Here's how the part is built. I have some questions about the finished solid (model axes, mm). A direction names the side the tool comes from. Give positions to 0.01 mm unless a question says otherwise; leave off trailing zeros. Loops run counter-clockwise (first coordinate to the right, second up) from the corner with the lowest first, then second, coordinate; pieces in that order, holes last. Notation, with made-up numbers: (-9, -14) - (6, -14) arc R29 ccw to (6, 11) - close; hole circle Ø9 at (-11.5, -6). An arc over 180 degrees is marked (long way). One line per item, written item: value. Start each with the question number.
```python
from build123d import *

# Parameters (mm, degrees)
F0_W          = 76.2
F0_H          = 38.1
F1_DEPTH      = 25.4
F2_R          = 11.1125
F3_DEPTH      = 12.7
F4_R          = 3.175
F5_DEPTH      = 38.101
F5_DEPTH_BACK = 139
F6_SIZE       = 3.175


# Not quite as in the source:
# - an extrude ends at something that could not be found from the text; its depth is read off the source's solid


with BuildPart() as f1:
    # F0 (on Top) → F1 (new body)
    with BuildSketch(Plane.XY):
        with Locations((38.1, -19.05)):
            Rectangle(F0_W, F0_H)
    extrude(amount=F1_DEPTH)

    # F2 (on face) → F3 (join)
    with BuildSketch(Plane.XY.offset(25.4)):
        with Locations((19.05, -19.05)):
            Circle(F2_R)
        with Locations((57.15, -19.05)):
            Circle(F2_R)
    extrude(amount=F3_DEPTH)

    # F4 (on face) → F5 (cut, two sides)
    with BuildSketch(Plane.XZ.offset(38.1)) as f5_sk:
        with Locations((38.1, 12.7)):
            Circle(F4_R)
    extrude(amount=-F5_DEPTH, mode=Mode.SUBTRACT)
    extrude(f5_sk.sketch, amount=F5_DEPTH_BACK, mode=Mode.SUBTRACT)

    # F6
    f6_edges = [f1.edges().sort_by_distance(p)[0] for p in [
        (46.0375, -19.05, 38.1),
        (7.9375, -19.05, 38.1),
        (38.1, -38.1, 25.4),
        (76.2, -19.05, 25.4),
        (38.1, 0, 25.4),
        (0, -19.05, 25.4),
    ]]
    chamfer(f6_edges, length=F6_SIZE)


solid = f1.part
```
(1) For faces 1 (the face through (29.65, -15.71, 30.1)), 2 (the face through (57, -19, 38.1)), which set-ups out of +Z, -Z, +X, -X, +Y, -Y let a thin tool reach every point of the face, with its end or its side?
(2) Please list where these lines run through material, in increasing order: probe 1 along Z at (x, y) = (38, -15); probe 2 along Z at (x, y) = (33.5, -24); probe 3 along X at (y, z) = (-11, 12). Write a range as from..to.
(3) If we section it at C-C on y = -5: List the corners of the cut face in (x, z) for me (3 decimals), plus the area to 3 significant figures.
(4) Will these pins go through, and if not, where does the flat tip stop? pin 1 (6 mm diameter, centred on x = 60.5, z = 27, fed in from +Y) (3 decimals); pin 2 (16 mm diameter, centred on x = 40.5, y = -16.5, fed in from +Z); pin 3 (3 mm diameter, centred on x = 20.5, z = 26, fed in from +Y) (3 decimals).
(5) If we section it at A-A on x = 38.1: List the corners of the cut face in (y, z) for me (3 decimals), plus the area to 3 significant figures.
(6) If we section it at D-D on x = 19.05: List the corners of the cut face in (y, z) for me (1 decimal).
(7) If we section it at B-B on z = 12.7: List the corners of the cut face in (x, y) for me (3 decimals), plus the area to 3 significant figures.
(8) If we mould it in two halves opening along X, with no side actions, what happens to faces 3 (the face through (19, -19, 38.1)), 4 (the face through (74.635, -19.317, 23.79)), 5 (the face through (67.75, -15.71, 30.1))? For each: pulls with the +X half, pulls with the -X half, needs draft (parallel to the pull), parting line crosses it, or undercut.
Found:
1. face 1: +Z
1. face 2: +Z, +X, -X, +Y, -Y
2. probe 1: 0..9.53, 15.87..25.4
2. probe 2: 0..25.4
2. probe 3: 0..35, 41.2..76.2
3. outline: (0, 0) - (76.2, 0) - (76.2, 22.225) - (73.025, 25.4) - (3.175, 25.4) - (0, 22.225) - close; hole circle Ø6.35 at (38.1, 12.7)
3. area: 1,890 mm^2
4. pin 1: y = -1.775
4. pin 2: z = 37.19
4. pin 3: y = -2.275
5. outline: (-38.1, 0) - (0, 0) - (0, 9.525) - (-38.1, 9.525) - close; (-38.1, 15.875) - (0, 15.875) - (0, 22.225) - (-3.175, 25.4) - (-34.925, 25.4) - (-38.1, 22.225) - close
5. area: 716 mm^2
6. outline: (-38.1, 0) - (0, 0) - (0, 22.2) - (-3.2, 25.4) - (-7.9, 25.4) - (-7.9, 34.9) - (-11.1, 38.1) - (-27, 38.1) - (-30.2, 34.9) - (-30.2, 25.4) - (-34.9, 25.4) - (-38.1, 22.2) - close
7. outline: (0, -38.1) - (34.925, -38.1) - (34.925, 0) - (0, 0) - close; (41.275, -38.1) - (76.2, -38.1) - (76.2, 0) - (41.275, 0) - close
7. area: 2,660 mm^2
8. face 3: needs draft
8. face 4: pulls with the +X half
8. face 5: undercut
